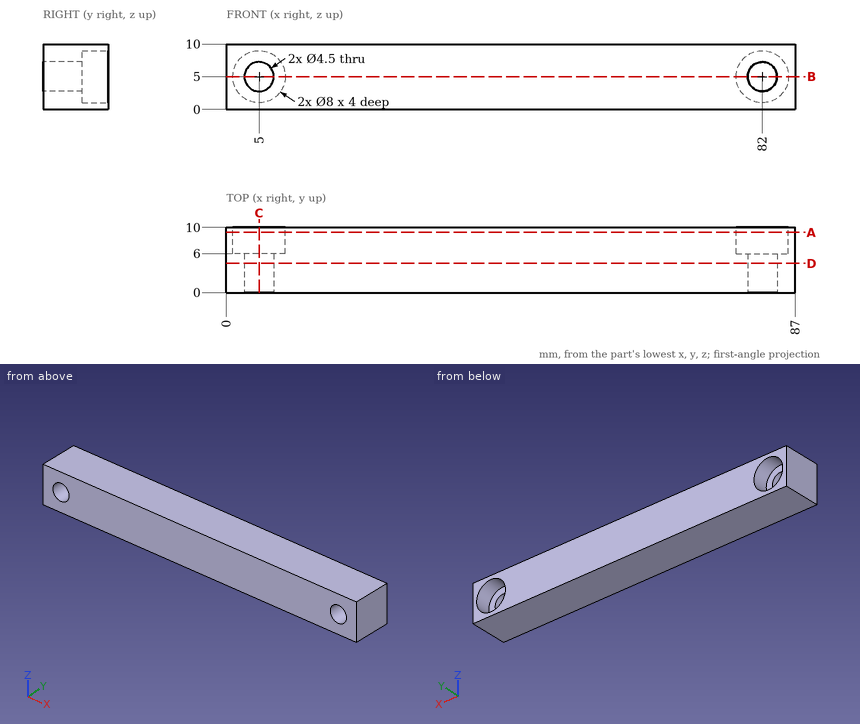
For this review, use the dimensioned drawing (mm, ordinates from the lowest corner) and the shaded views. Round coordinates to 2 decimals unless told otherwise and drop trailing zeros. Write each loop counter-clockwise with the first axis right and the second up, starting at its lowest first coordinate (ties: lowest second). Pieces come first, ordered by that corner, then holes. Notation, with made-up numbers: (-31, 25.5) - (-18, 25.5) arc R17 cw to (-18, 32.5) - close; hole circle Ø5 at (57.5, 73.5). An arc over 180 degrees is marked (long way). One line per item, written item: value. Start each with the question number.
1. Clearance check with flat-ended pins moving along their axes: P1, Ø4, axis at x = 4, z = 6.5, coming from the +Y side; P2, Ø6, axis at y = 8.5, z = 6.5, coming from the -X side; P3, Ø4, axis at x = 5, z = 5, coming from the +Y side. State where each tip first meets the part, or that it passes through.
2. Consider section A-A on y = 9.25. Write out the cut boundary in (x, z), and give its area (3 significant figures).
3. Consider section D-D on y = 4.5. Write out the cut boundary in (x, z).
4. Consider section B-B on z = 5. Write out the cut boundary in (x, y), and give its area (3 significant figures).
5. Consider section C-C on x = 5. Write out the cut boundary in (y, z), and give its area (3 significant figures).
6. To check wall thickness, follow L1, parallel to Z at x = 82, y = 8.1; L2, parallel to Z at x = 5, y = 4.1; L3, parallel to X at y = 1, z = 6.25. State the ranges of each line that lie inside material, in increasing order. Write a range as from..to.
Checks:
1. P1: stops at y = 6
1. P2: stops at x = 0
1. P3: passes through
2. outline: (0, 0) - (87, 0) - (87, 10) - (0, 10) - close; hole circle Ø8 at (5, 5); hole circle Ø8 at (82, 5)
2. area: 769 mm^2
3. outline: (0, 0) - (87, 0) - (87, 10) - (0, 10) - close; hole circle Ø4.5 at (5, 5); hole circle Ø4.5 at (82, 5)
4. outline: (0, 0) - (2.75, 0) - (2.75, 6) - (1, 6) - (1, 10) - (0, 10) - close; (7.25, 0) - (79.75, 0) - (79.75, 6) - (78, 6) - (78, 10) - (9, 10) - (9, 6) - (7.25, 6) - close; (84.25, 0) - (87, 0) - (87, 10) - (86, 10) - (86, 6) - (84.25, 6) - close
4. area: 752 mm^2
5. outline: (0, 0) - (10, 0) - (10, 1) - (6, 1) - (6, 2.75) - (0, 2.75) - close; (0, 7.25) - (6, 7.25) - (6, 9) - (10, 9) - (10, 10) - (0, 10) - close
5. area: 41.0 mm^2
6. L1: z = 0..1, 9..10
6. L2: z = 0..2.75, 7.25..10
6. L3: x = 0..3.13, 6.87..80.13, 83.87..87
